```python
from build123d import *

# Parameters (mm, degrees)
F0_W     = 50
F0_H     = 50
F0_R     = 4
F0_R_2   = 3
F0_R_3   = 1.5
F1_DEPTH = 30
F2_DEPTH = 6
F3_DEPTH = 6
F4_DEPTH = 11.5
F5_DEPTH = 3.5
F6_DEPTH = 6.5


with BuildPart() as f1:
    # F0 (on Front) → F1 (new body)
    with BuildSketch(Plane.XZ):
        Rectangle(F0_W, F0_H)
        with Locations((-15.5, -15.5)):
            Circle(F0_R, mode=Mode.SUBTRACT)
        with Locations((15.5, -15.5)):
            Circle(F0_R, mode=Mode.SUBTRACT)
        with Locations((-15.5, 15.5)):
            Circle(F0_R, mode=Mode.SUBTRACT)
        Circle(F0_R, mode=Mode.SUBTRACT)
        with Locations((15.5, 15.5)):
            Circle(F0_R, mode=Mode.SUBTRACT)
        with Locations((-15.5, 15.5)):
            Circle(F0_R)
        with Locations((-15.5, 15.5)):
            Circle(F0_R_2, mode=Mode.SUBTRACT)
        with Locations((-15.5, -15.5)):
            Circle(F0_R)
        with Locations((-15.5, -15.5)):
            Circle(F0_R_2, mode=Mode.SUBTRACT)
        with Locations((15.5, -15.5)):
            Circle(F0_R)
        with Locations((15.5, -15.5)):
            Circle(F0_R_2, mode=Mode.SUBTRACT)
        with Locations((15.5, 15.5)):
            Circle(F0_R)
        with Locations((15.5, 15.5)):
            Circle(F0_R_2, mode=Mode.SUBTRACT)
        with Locations((15.5, -15.5)):
            Circle(F0_R_2)
        with Locations((-15.5, -15.5)):
            Circle(F0_R_2)
        with Locations((15.5, 15.5)):
            Circle(F0_R_2)
        with Locations((-15.5, 15.5)):
            Circle(F0_R_2)
        Circle(F0_R)
        Circle(F0_R_3, mode=Mode.SUBTRACT)
        Circle(F0_R_3)
    extrude(amount=-F1_DEPTH)

    # F0 (on Front) → F2 (join)
    with BuildSketch(Plane.XZ):
        with Locations((-15.5, 15.5)):
            Circle(F0_R)
        with Locations((-15.5, 15.5)):
            Circle(F0_R_2, mode=Mode.SUBTRACT)
        with Locations((15.5, 15.5)):
            Circle(F0_R)
        with Locations((15.5, 15.5)):
            Circle(F0_R_2, mode=Mode.SUBTRACT)
        with Locations((15.5, -15.5)):
            Circle(F0_R)
        with Locations((15.5, -15.5)):
            Circle(F0_R_2, mode=Mode.SUBTRACT)
        with Locations((-15.5, -15.5)):
            Circle(F0_R)
        with Locations((-15.5, -15.5)):
            Circle(F0_R_2, mode=Mode.SUBTRACT)
    extrude(amount=F2_DEPTH)

    # F0 (on Front) → F3 (join)
    with BuildSketch(Plane.XZ):
        with Locations((-15.5, 15.5)):
            Circle(F0_R_2)
        with Locations((15.5, 15.5)):
            Circle(F0_R_2)
        with Locations((15.5, -15.5)):
            Circle(F0_R_2)
        with Locations((-15.5, -15.5)):
            Circle(F0_R_2)
    extrude(amount=F3_DEPTH)

    # F0 (on Front) → F4 (join)
    with BuildSketch(Plane.XZ):
        Circle(F0_R)
        Circle(F0_R_3, mode=Mode.SUBTRACT)
        Circle(F0_R_3)
    extrude(amount=F4_DEPTH)

    # F0 (on Front) → F5 (cut)
    with BuildSketch(Plane.XZ):
        with Locations((-15.5, -15.5)):
            Circle(F0_R)
        with Locations((-15.5, -15.5)):
            Circle(F0_R_2, mode=Mode.SUBTRACT)
        with Locations((15.5, -15.5)):
            Circle(F0_R)
        with Locations((15.5, -15.5)):
            Circle(F0_R_2, mode=Mode.SUBTRACT)
        with Locations((15.5, 15.5)):
            Circle(F0_R)
        with Locations((15.5, 15.5)):
            Circle(F0_R_2, mode=Mode.SUBTRACT)
        with Locations((-15.5, 15.5)):
            Circle(F0_R)
        with Locations((-15.5, 15.5)):
            Circle(F0_R_2, mode=Mode.SUBTRACT)
    extrude(amount=F5_DEPTH, mode=Mode.SUBTRACT)

    # F0 (on Front) → F6 (cut)
    with BuildSketch(Plane.XZ):
        Circle(F0_R)
        Circle(F0_R_3, mode=Mode.SUBTRACT)
    extrude(amount=F6_DEPTH, mode=Mode.SUBTRACT)


solid = f1.part
```
The listing builds one solid part. Answer for the finished solid, in the listing's coordinates (mm). A direction names the side the tool comes from. Round coordinates to 2 decimals unless told otherwise and drop trailing zeros. Order: outer loops, then holes, each group sorted by start corner. A loop starts at its lowest first (then second) coordinate and runs counter-clockwise, first axis right, second up. Notation, with made-up numbers: (23.5, 75) -> (41.5, 75) arc R10 ccw to (41.5, 92) -> close; hole circle Ø1 at (-6, 2.25). An arc over 180 degrees is marked (long way). Answer as CSV lines item,"result".
Q1. Which of the six approach directions +Z, -Z, +X, -X, +Y, -Y give full straight-line access (tool end or side, diameter ignored) to faces 5 (the cylindrical face through (13.1, -1.7, 13.7)), 6 (the flat face through (15, -6, -15)), 7 (the cylindrical face through (-18.45, -4.73, 18.2))?
Computed values:
face 5,"none"
face 6,"+Z, -Z, +X, -X, -Y"
face 7,"-Y"
Q2. Given pin 1 (2.5 mm diameter, centred on x = -14.5, z = -17, fed in from -Y); pin 2 (2 mm diameter, centred on x = 17.5, z = -5.5, fed in from -Y), each flat-ended and moving along its own axis, determine where each tip first touches the part or whether it passes through.
Computed values:
pin 1,"stops at y = -6"
pin 2,"stops at y = 0"
Q3. A cutting plane is placed at A-A on x = 0. Determine the outline of the cut face in (y, z).
Computed values:
outline,"(-11.5, -4) -> (-6.5, -4) -> (-6.5, -1.5) -> (0, -1.5) -> (0, -25) -> (30, -25) -> (30, 25) -> (0, 25) -> (0, 1.5) -> (-6.5, 1.5) -> (-6.5, 4) -> (-11.5, 4) -> close"
Q4. For a pull along X with two mould halves and no side action, classify faces 1 (the cylindrical face through (-0.867, -8.965, -3.905)), 2 (the cylindrical face through (-19.496, -4.732, -15.324)), 3 (the flat face through (25, 15, 0)), 4 (the flat face through (-16, -6, -15)) as +X half, -X half, draft (parallel to the pull), parting line (faces both ways), or undercut.
Computed values:
face 1,"parting line"
face 2,"undercut"
face 3,"+X half"
face 4,"draft"
Q5. A cutting plane is placed at C-C on y = -2. Determine the outline of the cut face in (x, z).
Computed values:
outline,"circle Ø6 at (-15.5, -15.5); circle Ø6 at (-15.5, 15.5); circle Ø3 at (0, 0); circle Ø6 at (15.5, -15.5); circle Ø6 at (15.5, 15.5)"
Q6. A cutting plane is placed at B-B on z = 15.5. Determine the outline of the cut face in (x, y), plus the area to 3 significant figures.
Computed values:
outline,"(-25, 0) -> (-18.5, 0) -> (-18.5, -3.5) -> (-19.5, -3.5) -> (-19.5, -6) -> (-11.5, -6) -> (-11.5, -3.5) -> (-12.5, -3.5) -> (-12.5, 0) -> (12.5, 0) -> (12.5, -3.5) -> (11.5, -3.5) -> (11.5, -6) -> (19.5, -6) -> (19.5, -3.5) -> (18.5, -3.5) -> (18.5, 0) -> (25, 0) -> (25, 30) -> (-25, 30) -> close"
area,"1,580 mm^2"
Q7. Consider line 1 (Y direction, x = 15, z = -19); line 2 (Y direction, x = -22, z = 18.5); line 3 (Y direction, x = -15, z = -17.5). Determine where each line is inside the solid, lowest interval first. Write a range as from..to.
Computed values:
line 1,"y = -6..-3.5, 0..30"
line 2,"y = 0..30"
line 3,"y = -6..30"
Q8. A cutting plane is placed at D-D on x = 15.5. Determine the outline of the cut face in (y, z).
Computed values:
outline,"(-6, -19.5) -> (-3.5, -19.5) -> (-3.5, -18.5) -> (0, -18.5) -> (0, -25) -> (30, -25) -> (30, 25) -> (0, 25) -> (0, 18.5) -> (-3.5, 18.5) -> (-3.5, 19.5) -> (-6, 19.5) -> (-6, 11.5) -> (-3.5, 11.5) -> (-3.5, 12.5) -> (0, 12.5) -> (0, -12.5) -> (-3.5, -12.5) -> (-3.5, -11.5) -> (-6, -11.5) -> close"
